```python
from build123d import *

# Parameters (mm, degrees)
SKETCH1_W               = 45
SKETCH1_H               = 45
BOSS_EXTRUDE1_DEPTH     = 15
CUT_EXTRUDE1_DEPTH      = 10
CUT_EXTRUDE2_DEPTH      = 38.243644172
CUT_EXTRUDE2_DEPTH_BACK = 38.243644172
SKETCH5_W               = 25
SKETCH5_H               = 25
BOSS_EXTRUDE2_DEPTH     = 20
FILLET1_R               = 3
SKETCH6_R               = 6
CUT_EXTRUDE4_DEPTH      = 28.99918
SKETCH7_W               = 13
SKETCH7_H               = 13
CUT_EXTRUDE5_DEPTH      = 13
FILLET2_R               = 3
CUT_EXTRUDE6_DEPTH      = 42.074189356
CUT_EXTRUDE6_DEPTH_BACK = 42.074189356
SKETCH8_R               = 1.5
SKETCH9_W               = 10.3
SKETCH9_H               = 10.3
CUT_EXTRUDE7_DEPTH      = 2.7
SKETCH10_R              = 6.85
BOSS_EXTRUDE3_DEPTH     = 2.3
CUT_EXTRUDE8_DEPTH      = 46.142818825
CUT_EXTRUDE9_DEPTH      = 46.142818825
CUT_EXTRUDE9_DEPTH_BACK = 46.142818825
SKETCH12_R              = 1.5


with BuildPart() as part:
    # Sketch1 → Boss-Extrude1 (new body)
    with BuildSketch(Plane(origin=(0, 0, 0), x_dir=(1, 0, 0), z_dir=(0, 1, 0))):
        with Locations((0.699698795, 4.865361446)):
            Rectangle(SKETCH1_W, SKETCH1_H)
    extrude(amount=BOSS_EXTRUDE1_DEPTH)

    # Sketch2 → Cut-Extrude1 (cut)
    with BuildSketch(Plane.XZ):
        Polygon((-21.800301205, 17.634638554), (-11.800301205, 17.634638554), (-11.800301205, -17.365361446), (23.199698795, -17.365361446), (23.199698795, -27.365361446), (-21.800301205, -27.365361446), align=None)
    extrude(amount=-CUT_EXTRUDE1_DEPTH, mode=Mode.SUBTRACT)

    # Sketch3 → Cut-Extrude2 (cut, two sides: drawn at the far end of the back side and taken through both)
    with BuildSketch(Plane.XZ.offset(-10).offset(-CUT_EXTRUDE2_DEPTH_BACK)):
        with BuildLine():
            Line((-11.340301205, -27.365361446), (12.739698795, -27.365361446))
            ThreePointArc((12.739698795, -27.365361446), (0.699698795, -22.366961339), (-11.340301205, -27.365361446))
        make_face()
        with BuildLine():
            Line((-21.800301205, 7.174638554), (-21.800301205, -16.905361446))
            ThreePointArc((-21.800301205, -16.905361446), (-16.801901098, -4.865361446), (-21.800301205, 7.174638554))
        make_face()
    extrude(amount=CUT_EXTRUDE2_DEPTH + CUT_EXTRUDE2_DEPTH_BACK, mode=Mode.SUBTRACT)

    # Sketch5 → Boss-Extrude2 (add)
    with BuildSketch(Plane(origin=(0, 15, 0), x_dir=(1, 0, 0), z_dir=(0, 1, 0))):
        with Locations((0.699698795, 4.865361446)):
            Rectangle(SKETCH5_W, SKETCH5_H)
    extrude(amount=BOSS_EXTRUDE2_DEPTH)

    # Fillet1
    fillet1_edges = [part.edges().sort_by_distance(p)[0] for p in [
        (-11.800301205, 25, -17.365361446),
        (-11.800301205, 25, 7.634638554),
        (13.199698795, 25, 7.634638554),
        (13.199698795, 25, -17.365361446),
        (-11.800301205, 35, -4.865361446),
        (0.699698795, 35, 7.634638554),
        (13.199698795, 35, -4.865361446),
        (0.699698795, 35, -17.365361446),
    ]]
    fillet(fillet1_edges, radius=FILLET1_R)

    # Sketch6 → Cut-Extrude4 (cut)
    with BuildSketch(Plane(origin=(0, 0, 0), x_dir=(-1, 0, 0), z_dir=(0, -1, 0))):
        with Locations(Location((-0.699698795, 4.865361446, 0), (0, 0, 90))):
            Circle(SKETCH6_R)
    extrude(amount=-CUT_EXTRUDE4_DEPTH, mode=Mode.SUBTRACT)

    # Sketch7 → Cut-Extrude5 (cut)
    with BuildSketch(Plane.XZ.offset(-28.99918)):
        with Locations((0.699698795, -4.865361446)):
            Rectangle(SKETCH7_W, SKETCH7_H)
    extrude(amount=CUT_EXTRUDE5_DEPTH, mode=Mode.SUBTRACT)

    # Fillet2
    fillet2_edges = [part.edges().sort_by_distance(p)[0] for p in [
        (-5.800301205, 28.99918, -4.865361446),
        (-5.800301205, 22.49918, 1.634638554),
        (0.699698795, 28.99918, -11.365361446),
        (-5.800301205, 22.49918, -11.365361446),
        (7.199698795, 28.99918, -4.865361446),
        (7.199698795, 22.49918, -11.365361446),
        (0.699698795, 28.99918, 1.634638554),
        (7.199698795, 22.49918, 1.634638554),
    ]]
    fillet(fillet2_edges, radius=FILLET2_R)

    # Sketch8 → Cut-Extrude6 (cut, two sides: drawn at the far end of the back side and taken through both)
    with BuildSketch(Plane(origin=(0, 15, 0), x_dir=(1, 0, 0), z_dir=(0, 1, 0)).offset(-CUT_EXTRUDE6_DEPTH_BACK)):
        with Locations(Location((-16.800301205, 22.365361446, 0), (0, 0, 270))):
            Circle(SKETCH8_R)
        with Locations(Location((18.199698795, 22.365361446, 0), (0, 0, 270))):
            Circle(SKETCH8_R)
        with Locations(Location((18.199698795, -12.634638554, 0), (0, 0, 270))):
            Circle(SKETCH8_R)
        with Locations(Location((-16.800301205, -12.634638554, 0), (0, 0, 270))):
            Circle(SKETCH8_R)
    extrude(amount=CUT_EXTRUDE6_DEPTH + CUT_EXTRUDE6_DEPTH_BACK, mode=Mode.SUBTRACT)

    # Sketch9 → Cut-Extrude7 (cut)
    with BuildSketch(Plane(origin=(0, 15, 0), x_dir=(1, 0, 0), z_dir=(0, 1, 0))):
        with Locations((-16.650301205, 22.215361446)):
            Rectangle(SKETCH9_W, SKETCH9_H)
    extrude(amount=-CUT_EXTRUDE7_DEPTH, mode=Mode.SUBTRACT)

    # Sketch10 → Boss-Extrude3 (add)
    with BuildSketch(Plane.XZ.offset(-10)):
        with Locations((-16.800301205, -22.365361446)):
            Circle(SKETCH10_R)
    extrude(amount=-BOSS_EXTRUDE3_DEPTH)

    # Sketch11 → Cut-Extrude8 (cut, through all)
    with BuildSketch(Plane.XZ.offset(-10)):
        with BuildLine():
            Line((-21.482448148, -27.365361446), (-21.800301205, -27.365361446))
            Line((-21.800301205, -27.365361446), (-21.800301205, -27.047508389))
            ThreePointArc((-21.800301205, -27.047508389), (-21.650197676, -27.215257917), (-21.482448148, -27.365361446))
        make_face()
    extrude(amount=-CUT_EXTRUDE8_DEPTH, mode=Mode.SUBTRACT)

    # Sketch12 → Cut-Extrude9 (cut, two sides: drawn at the far end of the back side and taken through both)
    with BuildSketch(Plane.XZ.offset(-10).offset(-CUT_EXTRUDE9_DEPTH_BACK)):
        with Locations(Location((-17.110205033, -22.675265274, 0), (0, 0, 90))):
            Circle(SKETCH12_R)
    extrude(amount=CUT_EXTRUDE9_DEPTH + CUT_EXTRUDE9_DEPTH_BACK, mode=Mode.SUBTRACT)


solid = part.part
```
The listing builds one solid part. Answer for the finished solid, in the listing's coordinates (mm). A direction names the side the tool comes from. Round coordinates to 2 decimals unless told otherwise and drop trailing zeros. Loops run counter-clockwise (first coordinate to the right, second up) from the corner with the lowest first, then second, coordinate; pieces in that order, holes last. Notation, with made-up numbers: (-10.75, 76.5) - (37.25, 76.5) arc R33 cw to (37.25, 115.5) - close; hole circle Ø8 at (18, -23.75). An arc over 180 degrees is marked (long way). Return JSON: item names as keys, results as strings. Group by question number.
1. The part is cut by section C-C on x = 12. Determine the outline of the cut face in (y, z), then the cut area to 3 significant figures.
2. The part is cut by section D-D on y = 8. Determine the outline of the cut face in (x, z), then the cut area to 3 significant figures.
3. The mould has two halves that part along Z. Classify faces 6 (the flat face through (18, 12, -27.365)), 7 (the flat face through (5, 7, 17.635)), 8 (the flat face through (-5, 10, -18)), 9 (the flat face through (-1, 15.999, -11)): pulls with the +Z half, pulls with the -Z half, needs draft (parallel to the pull), parting line crosses it, or undercut.
4. The part is cut by section A-A on y = 28. Determine the outline of the cut face in (x, z).
5. Which of the six approach directions +Z, -Z, +X, -X, +Y, -Y give full straight-line access (tool end or side, diameter ignored) to faces 1 (the flat face through (1, 23, 7.635)), 2 (the flat face through (-17, 14, -17.065)), 3 (the cylindrical face through (-4.94, 28.1, -4.82)), 4 (the flat face through (-11.8, 5, 0)), 5 (the cylindrical face through (12.298, 23.619, 6.779))?
6. Consider probe 1 along Z at (x, y) = (-2.5, 19.5); probe 2 along X at (y, z) = (24.5, -10); probe 3 along Y at (x, z) = (14, -19). Determine where each line is inside the solid, lowest interval first.
7. Each of these flat-tipped pins is pushed along its axis until it touches: P1, Ø2.5, axis at x = 16, y = 12, coming from the -Z side; P2, Ø4, axis at x = 0, y = 9.5, coming from the -Z side; P3, Ø18.5, axis at x = 4, y = 23.5, coming from the -Z side; P4, Ø2.5, axis at x = -17.11, z = -22.68, coming from the +Y side. Where does it stop, or does it pass through?
8. The part is cut by section B-B on z = -26. Determine the outline of the cut face in (x, y).
Resolved:
{
 "1": {"outline": "(0, -17.37) - (10, -17.37) - (10, -26.67) - (15, -26.67) - (15, -16.77) - (32, -16.77) arc R2.4 ccw to (34.4, -14.37) - (34.4, 4.63) arc R2.4 ccw to (32, 7.03) - (15, 7.03) - (15, 17.63) - (0, 17.63) - close", "area": "1,030 mm²"},
 "2": {"outline": "(-11.8, -17.37) - (23.2, -17.37) - (23.2, 17.63) - (-11.8, 17.63) - close; hole circle Ø12 at (0.7, -4.87); hole circle Ø3 at (18.2, 12.63)", "area": "1,100 mm²"},
 "3": {"face 6": "pulls with the -Z half", "face 7": "pulls with the +Z half", "face 8": "needs draft", "face 9": "undercut"},
 "4": {"outline": "(-11.8, -14.37) arc R3 ccw to (-8.8, -17.37) - (10.2, -17.37) arc R3 ccw to (13.2, -14.37) - (13.2, 4.63) arc R3 ccw to (10.2, 7.63) - (-8.8, 7.63) arc R3 ccw to (-11.8, 4.63) - close; hole (-5.04, -8.37) arc R2.24 ccw to (-2.8, -10.6) - (4.2, -10.6) arc R2.24 ccw to (6.44, -8.37) - (6.44, -1.37) arc R2.24 ccw to (4.2, 0.87) - (-2.8, 0.87) arc R2.24 ccw to (-5.04, -1.37) - close"},
 "5": {"face 1": "+Z, +X, -X, +Y", "face 2": "-Z, -X, +Y", "face 3": "none", "face 4": "+Z, -Z, -X, -Y", "face 5": "+Z, +X, +Y"},
 "6": {"probe 1": "z = -17.37 to -11.37, 1.63 to 7.63", "probe 2": "x = -11.8 to -5.32, 6.72 to 13.2", "probe 3": "y = 10 to 15"},
 "7": {"P1": "stops at z = -27.37", "P2": "stops at z = -22.57", "P3": "stops at z = -23.85", "P4": "passes through"},
 "8": {"outline": "(-22.61, 10) - (-9.8, 10) - (-9.8, 15) - (-11.5, 15) - (-11.5, 12.3) - (-22.61, 12.3) - close; (11.2, 10) - (23.2, 10) - (23.2, 15) - (11.2, 15) - close"}
}
